Input: part model. Units: mm. Frame: model coordinates. A direction names the side the tool comes from. Round coordinates to 2 decimals unless told otherwise and drop trailing zeros. Loops run counter-clockwise (first coordinate to the right, second up) from the corner with the lowest first, then second, coordinate; pieces in that order, holes last.
(1) Cut plane A-A, the plane y = 13.75. Output: boundary loops of the cut face in (x, z), and give its area (3 significant figures).
(2) Draft query along X for faces 1 (the face through (15, 13, 22)), 2 (the face through (-26.94, 12.52, -19.62)), 3 (the face through (0, 25.4, 8)). Return one class per face: released by +X, released by -X, zero draft, split by the parting line, or undercut.
(3) Cut plane B-B, the plane z = -21. Output: boundary loops of the cut face in (x, y).
(4) Line query: line 1 (X direction, y = 8, z = 16); line 2 (X direction, y = 8.5, z = -9); line 3 (Z direction, x = 43, y = 24.25). Output: solid intervals per line, ascending.
(5) Access query for faces 4 (the face through (-15, 13, 23)), 5 (the face through (26.54, 12.52, -19.22)), 6 (the face through (0, 0, 8)). Directions: +Z, -Z, +X, -X, +Y, -Y. A direction counts if a zero-diameter tool reaches every point of the face in a straight line with its end or side. Return the directions, or none.
(6) Cut plane C-C, the plane x = 0. Output: boundary loops of the cut face in (y, z).
(7) First-contact query: pin 1 Ø1 at (y, z) = (5, 36.5) entering from -X; pin 2 Ø12 at (x, z) = (-16.5, 4) entering from -Y; pin 3 Ø12 at (x, y) = (26, 18.5) entering from +Z; pin 4 Ø7.5 at (x, y) = (6, 16.5) entering from -Z. Flat tips, straight axial feed; report the tip coordinate or a pass-through.
(8) Cut plane D-D, the plane z = 32. Output: boundary loops of the cut face in (x, y).
from build123d import *

# Parameters (mm, degrees)
F0_R     = 12.5
F1_DEPTH = 25.4


with BuildPart() as f1:
    # F0 (on Front) → F1 (new body)
    with BuildSketch(Plane.XZ):
        with BuildLine():
            Line((15, 10), (15, 35))
            ThreePointArc((15, 35), (0, 50), (-15, 35))
            Line((-15, 35), (-15, 10))
            Line((-15, 10), (-50, -25))
            Line((-50, -25), (-41.1611652352, -33.8388347648))
            Line((-41.1611652352, -33.8388347648), (-12.3223304703, -5))
            Line((-12.3223304703, -5), (0, -5))
            Line((0, -5), (12.3223304703, -5))
            Line((12.3223304703, -5), (41.1611652352, -33.8388347648))
            Line((41.1611652352, -33.8388347648), (50, -25))
            Line((50, -25), (15, 10))
        make_face()
        with Locations((0, 35)):
            Circle(F0_R, mode=Mode.SUBTRACT)
        with Locations((0, 35)):
            Circle(F0_R)
    extrude(amount=-F1_DEPTH)


solid = f1.part
Reported:
1. outline: (-50, -25) - (-41.16, -33.84) - (-12.32, -5) - (12.32, -5) - (41.16, -33.84) - (50, -25) - (15, 10) - (15, 35) arc R15 ccw to (-15, 35) - (-15, 10) - close
1. area: 2,640 mm2
2. face 1: released by +X
2. face 2: undercut
2. face 3: zero draft
3. outline: (-46, 0) - (-28.32, 0) - (-28.32, 25.4) - (-46, 25.4) - close; (28.32, 0) - (46, 0) - (46, 25.4) - (28.32, 25.4) - close
4. line 1: x = -15 to 15
4. line 2: x = -34 to -16.32, 16.32 to 34
4. line 3: z = -32 to -18
5. face 4: +Z, -X, +Y, -Y
5. face 5: -Z, +Y, -Y
5. face 6: +Z, -Z, +X, -X, -Y
6. outline: (0, -5) - (25.4, -5) - (25.4, 50) - (0, 50) - close
7. pin 1: stops at x = -14.97
7. pin 2: stops at y = 0
7. pin 3: stops at z = 5
7. pin 4: stops at z = -5
8. outline: (-15, 0) - (15, 0) - (15, 25.4) - (-15, 25.4) - close
